```python
from build123d import *

# Parameters (mm, degrees)
SKETCH1_R           = 1.5
SKETCH1_R_2         = 6
BOSS_EXTRUDE1_DEPTH = 3


with BuildPart() as part:
    # Sketch1 → Boss-Extrude1 (new body)
    with BuildSketch(Plane(origin=(0, 0, 0), x_dir=(1, 0, 0), z_dir=(0, 1, 0))):
        with BuildLine():
            Line((-11.47745757, -9.657534247), (-2.486782474, -20.342465753))
            ThreePointArc((-2.486782474, -20.342465753), (0, -21.5), (2.486782474, -20.342465753))
            Line((2.486782474, -20.342465753), (11.47745757, -9.657534247))
            ThreePointArc((11.47745757, -9.657534247), (15, 0), (11.47745757, 9.657534247))
            Line((11.47745757, 9.657534247), (2.486782474, 20.342465753))
            ThreePointArc((2.486782474, 20.342465753), (0, 21.5), (-2.486782474, 20.342465753))
            Line((-2.486782474, 20.342465753), (-11.47745757, 9.657534247))
            ThreePointArc((-11.47745757, 9.657534247), (-15, 0), (-11.47745757, -9.657534247))
        make_face()
        with Locations((0, -18.25)):
            Circle(SKETCH1_R, mode=Mode.SUBTRACT)
        Circle(SKETCH1_R_2, mode=Mode.SUBTRACT)
        with Locations((0, 18.25)):
            Circle(SKETCH1_R, mode=Mode.SUBTRACT)
    extrude(amount=BOSS_EXTRUDE1_DEPTH)


solid = part.part
```
Work out the finished part from the listing and answer in its coordinate system (mm). Round coordinates to 2 decimals unless told otherwise and drop trailing zeros. Write each loop counter-clockwise with the first axis right and the second up, starting at its lowest first coordinate (ties: lowest second). Pieces come first, ordered by that corner, then holes.
1) A cutting plane is placed at D-D on z = -18.25. Determine the outline of the cut face in (x, y).
2) Consider probe 1 along Z at (x, y) = (0, 0.9); probe 2 along Z at (x, y) = (-1, 1.7); probe 3 along X at (y, z) = (1.9, 18.25). Determine where each line is inside the solid, lowest interval first.
3) A cutting plane is placed at C-C on x = 0. Determine the outline of the cut face in (y, z).
4) Flat-ended cylindrical pins translate along their axes: P1, Ø1.5, axis at x = 1.5, y = 1, coming from the +Z side; P2, Ø11, axis at x = 0, z = 0, coming from the +Y side. Find the tip coordinate at first contact, or state that the pin passes through.
5) Determine the mould class of faces 1 (the face through (-7.045, 1.479, 14.925)), 2 (the face through (15, 1, 0)), 3 (the face through (-0.195, 1.479, -19.737)) for opening direction X: pulls with the +X half, pulls with the -X half, needs draft (parallel to the pull), parting line crosses it, or undercut.
6) A cutting plane is placed at B-B on y = 1.5. Determine the outline of the cut face in (x, z), and give its area (3 significant figures).
7) A cutting plane is placed at A-A on z = 0. Determine the outline of the cut face in (x, y).
Entries:
1. outline: (-4.25, 0) - (-1.5, 0) - (-1.5, 3) - (-4.25, 3) - close; (1.5, 0) - (4.25, 0) - (4.25, 3) - (1.5, 3) - close
2. probe 1: z = -21.5 to -19.75, -16.75 to -6, 6 to 16.75, 19.75 to 21.5
2. probe 2: z = -21.34 to -19.37, -17.13 to -5.92, 5.92 to 17.13, 19.37 to 21.34
2. probe 3: x = -4.25 to -1.5, 1.5 to 4.25
3. outline: (0, -21.5) - (3, -21.5) - (3, -19.75) - (0, -19.75) - close; (0, -16.75) - (3, -16.75) - (3, -6) - (0, -6) - close; (0, 6) - (3, 6) - (3, 16.75) - (0, 16.75) - close; (0, 19.75) - (3, 19.75) - (3, 21.5) - (0, 21.5) - close
4. P1: stops at z = 21.41
4. P2: passes through
5. face 1: pulls with the -X half
5. face 2: pulls with the +X half
5. face 3: undercut
6. outline: (-11.48, -9.66) - (-2.49, -20.34) arc R3.25 ccw to (2.49, -20.34) - (11.48, -9.66) arc R15 ccw to (11.48, 9.66) - (2.49, 20.34) arc R3.25 ccw to (-2.49, 20.34) - (-11.48, 9.66) arc R15 ccw to start; hole circle Ø12 at (0, 0); hole circle Ø3 at (0, -18.25); hole circle Ø3 at (0, 18.25)
6. area: 716 mm2
7. outline: (-15, 0) - (-6, 0) - (-6, 3) - (-15, 3) - close; (6, 0) - (15, 0) - (15, 3) - (6, 3) - close
